from build123d import *

# Parameters (mm, degrees)
BOSS_EXTRUDE1_DEPTH = 27.775
SKETCH2_R           = 27.5
BOSS_EXTRUDE2_DEPTH = 20.55
SKETCH3_R           = 10
SKETCH3_R_2         = 6
EXTRUDE_THIN1_DEPTH = 8
SKETCH4_R           = 6
CUT_EXTRUDE2_DEPTH  = 11.8
SKETCH5_W           = 20
SKETCH5_H           = 5
BOSS_EXTRUDE3_DEPTH = 8


with BuildPart() as part:
    # Sketch1 → Boss-Extrude1 (new, symmetric)
    with BuildSketch(Plane.XY):
        Polygon((-58.75, 0), (58.75, 0), (58.75, 85), (82.55, 85), (82.55, 96.8), (58.75, 96.8), (58.75, 116.65), (-58.75, 116.65), (-58.75, 96.8), (-82.55, 96.8), (-82.55, 85), (-58.75, 85), align=None)
    extrude(amount=BOSS_EXTRUDE1_DEPTH, both=True)

    # Sketch2 → Boss-Extrude2 (add)
    with BuildSketch(Plane(origin=(0, 116.65, 0), x_dir=(1, 0, 0), z_dir=(0, 1, 0))):
        with BuildLine():
            Line((19.756400184, 5.711832399), (7.756400184, 5.711832399))
            ThreePointArc((7.756400184, 5.711832399), (8.205780532, 2.871615204), (8.356121921, 0))
            ThreePointArc((8.356121921, 0), (8.205780532, -2.871615204), (7.756400184, -5.711832399))
            Line((7.756400184, -5.711832399), (19.756400184, -5.711832399))
            ThreePointArc((19.756400184, -5.711832399), (25.468232583, 0), (19.756400184, 5.711832399))
        make_face()
        with Locations((-19.143878079, 0)):
            Circle(SKETCH2_R)
    extrude(amount=BOSS_EXTRUDE2_DEPTH)

    # Sketch3 → Extrude-Thin1 (add)
    with BuildSketch(Plane(origin=(0, 137.2, 0), x_dir=(1, 0, 0), z_dir=(0, 1, 0))):
        with Locations((-19.143878079, 0)):
            Circle(SKETCH3_R)
        with Locations((-19.143878079, 0)):
            Circle(SKETCH3_R_2, mode=Mode.SUBTRACT)
    extrude(amount=EXTRUDE_THIN1_DEPTH)

    # Sketch4 → Cut-Extrude2 (cut)
    with BuildSketch(Plane(origin=(0, 96.8, 0), x_dir=(1, 0, 0), z_dir=(0, 1, 0))):
        with Locations(Location((67.475, 0, 0), (0, 0, 180))):
            Circle(SKETCH4_R)
        with Locations(Location((-67.475, 0, 0), (0, 0, 180))):
            Circle(SKETCH4_R)
    extrude(amount=-CUT_EXTRUDE2_DEPTH, mode=Mode.SUBTRACT)

    # Sketch5 → Boss-Extrude3 (add)
    with BuildSketch(Plane(origin=(58.75, 0, 0), x_dir=(0, 0, -1), z_dir=(1, 0, 0))):
        with Locations((0, 17.5)):
            Rectangle(SKETCH5_W, SKETCH5_H)
    boss_extrude3 = extrude(amount=BOSS_EXTRUDE3_DEPTH)

    # Mirror1: Boss-Extrude3 across plane
    add(boss_extrude3.mirror(Plane(origin=(0, 0, 0), x_dir=(0, 0, 1), z_dir=(1, 0, 0))))


solid = part.part
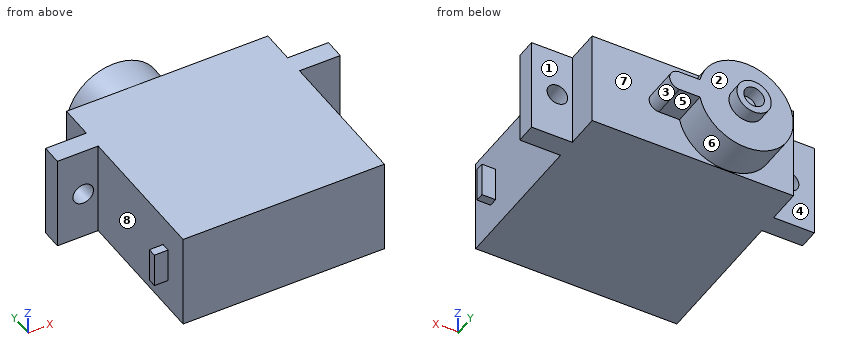
The model under review builds one solid part; all positions refer to its coordinate system, in mm. Face numbers are marked on the shaded views. A direction names the side the tool comes from. Round coordinates to 2 decimals unless told otherwise and drop trailing zeros. Loops run counter-clockwise (first coordinate to the right, second up) from the corner with the lowest first, then second, coordinate; pieces in that order, holes last. Notation, with made-up numbers: M 84.25,-2 L 124.25,-2 A25 ccw 124.25,23 Z; hole C -38,58 d4. An arc over 180 degrees is marked long. Answer as a JSON object with one key per item and string values.
Item 1: We need section D-D, the plane z = 8. State the section outline as (x, y) points, and give its area (3 significant figures).
Check sheet entries:
{"outline": "M -82.55,85 L -58.75,85 L -58.75,20 L -66.75,20 L -66.75,15 L -58.75,15 L -58.75,0 L 58.75,0 L 58.75,15 L 66.75,15 L 66.75,20 L 58.75,20 L 58.75,85 L 82.55,85 L 82.55,96.8 L 58.75,96.8 L 58.75,116.65 L 7.17,116.65 L 7.17,137.2 L -13.14,137.2 L -13.14,145.2 L -25.14,145.2 L -25.14,137.2 L -45.45,137.2 L -45.45,116.65 L -58.75,116.65 L -58.75,96.8 L -82.55,96.8 Z", "area": "15,500 mm2"}
Item 2: Clearance check with flat-ended pins moving along their axes: P1, Ø4, axis at x = 64.5, z = 3, coming from the -Y side; P2, Ø1, axis at y = 125, z = 0, coming from the +X side; P3, Ø2.5, axis at y = 17.5, z = -3, coming from the -X side; P4, Ø12, axis at x = -4.5, z = 17, coming from the -Y side. State where each tip first meets the part, or that it passes through.
Check sheet entries:
{"P1": "y = 15", "P2": "x = 25.47", "P3": "x = -66.75", "P4": "y = 0"}
Item 3: For line 1 along Y through (x, z) = (-60, -3); line 2 along X through (y, z) = (106, -12.5); line 3 along Y through (x, z) = (20.5, 23), list the stretches that pass through material, from the lowest coordinate up.
Check sheet entries:
{"line 1": "15 to 20, 85 to 96.8", "line 2": "-58.75 to 58.75", "line 3": "0 to 116.65"}
Item 4: Tool access review of the marked faces 1, 2, 3, 4 and 5: name each direction out of +Z, -Z, +X, -X, +Y, -Y from which nothing blocks a thin tool from reaching the whole face with its end or side.
Check sheet entries:
{"face 1": "+Z, -Z, +X, +Y", "face 2": "+Y", "face 3": "+X, +Y", "face 4": "+Z, -Z, -X, +Y", "face 5": "-Z, +X, +Y"}
Item 5: The part is to be moulded in two halves that separate along Y. For the marked faces 6, 7 and 8, say which applies: +Y half, -Y half, draft (parallel to the pull), parting line (faces both ways), or undercut.
Check sheet entries:
{"face 6": "draft", "face 7": "+Y half", "face 8": "undercut"}
Item 6: We need section C-C, the plane y = 43. State the section outline as (x, z) points (3 decimals).
Check sheet entries:
{"outline": "M -58.75,-27.775 L 58.75,-27.775 L 58.75,27.775 L -58.75,27.775 Z"}
Item 7: We need section A-A, the plane x = 11. State the section outline as (y, z) points (3 decimals).
Check sheet entries:
{"outline": "M 0,-27.775 L 116.65,-27.775 L 116.65,-5.712 L 137.2,-5.712 L 137.2,5.712 L 116.65,5.712 L 116.65,27.775 L 0,27.775 Z"}
Item 8: We need section B-B, the plane z = 0. State how many separate pieces and enclosed holes the cut face has, and give its area (3 significant figures).
Check sheet entries:
{"separate pieces": "3", "enclosed holes": "0", "area": "15,600 mm2"}
